The model under review builds one solid part; all positions refer to its coordinate system, in mm. A direction names the side the tool comes from. Coordinates: 2 decimals unless noted, no trailing zeros. Order: outer loops, then holes, each group sorted by start corner. A loop starts at its lowest first (then second) coordinate and runs counter-clockwise, first axis right, second up. Notation, with made-up numbers: (32.5, 53) - (69.5, 53) arc R34 ccw to (69.5, 86) - close; hole circle Ø4 at (-24.5, 11). An arc over 180 degrees is marked (long way). Answer in a Markdown table with one row per item.
```python
from build123d import *

# Parameters (mm, degrees)
SKETCH6_W           = 20
SKETCH6_H           = 16
BOSS_EXTRUDE5_DEPTH = 6
SKETCH7_W           = 10
SKETCH7_H           = 16
BOSS_EXTRUDE6_DEPTH = 8
SKETCH8_W           = 14.5
SKETCH8_H           = 16
BOSS_EXTRUDE7_DEPTH = 13
SKETCH9_R           = 5
CUT_EXTRUDE1_DEPTH  = 32.890437438
FILLET1_R           = 7.5
FILLET2_R           = 7.5


with BuildPart() as part:
    # Sketch6 → Boss-Extrude5 (new body)
    with BuildSketch(Plane(origin=(0, 0, 0), x_dir=(1, 0, 0), z_dir=(0, 1, 0))):
        with Locations((10, 8)):
            Rectangle(SKETCH6_W, SKETCH6_H)
    extrude(amount=BOSS_EXTRUDE5_DEPTH)

    # Sketch7 → Boss-Extrude6 (add)
    with BuildSketch(Plane.XZ):
        with Locations((10, -8)):
            Rectangle(SKETCH7_W, SKETCH7_H)
    extrude(amount=BOSS_EXTRUDE6_DEPTH)

    # Sketch8 → Boss-Extrude7 (add)
    with BuildSketch(Plane(origin=(0, 6, 0), x_dir=(1, 0, 0), z_dir=(0, 1, 0))):
        with Locations((10, 8)):
            Rectangle(SKETCH8_W, SKETCH8_H)
    extrude(amount=BOSS_EXTRUDE7_DEPTH)

    # Sketch9 → Cut-Extrude1 (cut, through all)
    with BuildSketch(Plane.XY):
        with Locations((10, 11)):
            Circle(SKETCH9_R)
    extrude(amount=-CUT_EXTRUDE1_DEPTH, mode=Mode.SUBTRACT)

    # Fillet1
    # the kernel refuses this fillet: 7.5 mm, written as the material it takes off along each edge
    with BuildSketch(Plane(origin=(17.25, 19, -34.75), x_dir=(-1, 0, 0), z_dir=(0, 0, 1))) as fillet1_piece_1:
        with BuildLine():
            CenterArc((FILLET1_R, FILLET1_R), FILLET1_R, 180, 90)
            Line((0, FILLET1_R), (0, 0))
            Line((0, 0), (FILLET1_R, 0))
        make_face()
    extrude(amount=53.5, mode=Mode.SUBTRACT)
    with BuildSketch(Plane(origin=(2.75, 19, 18.75), x_dir=(0, -1, 0), z_dir=(0, 0, -1))) as fillet1_piece_2:
        with BuildLine():
            CenterArc((FILLET1_R, -FILLET1_R), FILLET1_R, 90, 90)
            Line((0, -FILLET1_R), (0, 0))
            Line((0, 0), (FILLET1_R, 0))
        make_face()
    extrude(amount=53.5, mode=Mode.SUBTRACT)

    # Fillet2
    # the kernel refuses this fillet: 7.5 mm, written as the material it adds along each edge
    with BuildSketch(Plane(origin=(17.25, 6, -16), x_dir=(1, 0, 0), z_dir=(0, 0, 1))) as fillet2_piece_1:
        with BuildLine():
            CenterArc((7.496865043, 5.806657581), FILLET2_R, 181.171427285, 49.563032728)
            Line((-0.001567478, 5.65332879), (-0.75141073, 5.637995911))
            ThreePointArc((-0.75141073, 5.637995911), (-0.75, 5.5), (-0.75, 0))
            Line((-0.75, 0), (0, -0.75))
            ThreePointArc((0, -0.75), (1.375, -0.75), (2.275313496, -0.580665758))
            Line((2.275313496, -0.580665758), (2.75, 0))
        make_face()
    extrude(amount=16)
    with BuildSketch(Plane(origin=(2.75, 6, 0), x_dir=(0.00027726642617420565, 0.9999999615616638, 0), z_dir=(0, 0, -1))) as fillet2_piece_2:
        with BuildLine():
            CenterArc((5.804578729, -7.498474746), FILLET2_R, 91.155541089, 49.563032728)
            Line((-0.000762483, -2.749999894), (-0.581296604, -2.275152409))
            ThreePointArc((-0.581296604, -2.275152409), (-0.750381213, -1.374791997), (-0.749999971, 0.00020795))
            Line((-0.749999971, 0.00020795), (0.00020795, 0.749999971))
            ThreePointArc((0.00020795, 0.749999971), (5.500207738, 0.748475006), (5.638204036, 0.749847475))
            Line((5.638204036, 0.749847475), (5.653329008, 0))
        make_face()
    extrude(amount=16)


solid = part.part
```
Item 1: We need section C-C, the plane y = 11. Write out the cut boundary in (x, z), then the cut area to 3 significant figures.
Check values:
| item | result |
|---|---|
| outline | (2.71, -16) - (5, -16) - (5, 0) - (2.71, 0) - close; (15, -16) - (17.29, -16) - (17.29, 0) - (15, 0) - close |
| area | 73.3 mm^2 |
Item 2: Mouldability with a two-part tool opening along X and no side actions: class faces 1 (the face through (20, 3, -8)), 2 (the face through (17, 0, -8)), 3 (the face through (14.77, 12.5, -7.89)) as +X half, -X half, draft (parallel to the pull), parting line (faces both ways), or undercut.
Check values:
| item | result |
|---|---|
| face 1 | +X half |
| face 2 | draft |
| face 3 | undercut |
Item 3: We need section B-B, the plane x = 13.25. Write out the cut boundary in (y, z).
Check values:
| item | result |
|---|---|
| outline | (-8, -16) - (7.2, -16) - (7.2, 0) - (-8, 0) - close; (14.8, -16) - (18.13, -16) - (18.13, 0) - (14.8, 0) - close |
Item 4: We need section D-D, the plane y = -5. Write out the cut boundary in (x, z), then the cut area to 3 significant figures.
Check values:
| item | result |
|---|---|
| outline | (5, -16) - (15, -16) - (15, 0) - (5, 0) - close |
| area | 160 mm^2 |
Item 5: We need section A-A, the plane z = -8.75. Write out the cut boundary in (x, y).
Check values:
| item | result |
|---|---|
| outline | (0, 0) - (5, 0) - (5, -8) - (15, -8) - (15, 0) - (20, 0) - (20, 6) arc R7.5 cw to (17.25, 11.65) arc R7.5 ccw to (10, 19) arc R7.5 ccw to (2.75, 11.65) arc R7.5 cw to (0, 6) - close; hole circle Ø10 at (10, 11) |
Item 6: Clearance check with flat-ended pins moving along their axes: pin 1 Ø2.5 at (x, z) = (17.5, -11) entering from -Y; pin 2 Ø4 at (y, z) = (-4.5, -11.5) entering from +X; pin 3 Ø1.5 at (x, z) = (8.5, -8) entering from +Y; pin 4 Ø6 at (x, y) = (10, 11) entering from -Z. State where each tip first meets the part, or that it passes through.
Check values:
| item | result |
|---|---|
| pin 1 | y = 0 |
| pin 2 | x = 15 |
| pin 3 | y = 18.93 |
| pin 4 | through |
Item 7: Tool access review of faces 4 (the face through (5, -4, -8)), 5 (the face through (15, -4, -8)), 6 (the face through (0, 3, -8)): name each direction out of +Z, -Z, +X, -X, +Y, -Y from which nothing blocks a thin tool from reaching the whole face with its end or side.
Check values:
| item | result |
|---|---|
| face 4 | +Z, -Z, -X, -Y |
| face 5 | +Z, -Z, +X, -Y |
| face 6 | +Z, -Z, -X, +Y, -Y |
Item 8: To check wall thickness, follow line 1 (Y direction, x = 10, z = -12.5); line 2 (X direction, y = -2.25, z = -8.25); line 3 (Y direction, x = 9.25, z = -6.75). State the ranges of each line that lie inside material, in increasing order. Write a range as from..to.
Check values:
| item | result |
|---|---|
| line 1 | -8..6, 16..19 |
| line 2 | 5..15 |
| line 3 | -8..6.06, 15.94..18.93 |
